from build123d import *

# Parameters (mm, degrees)
SKETCH_1_R               = 20
EXTRUDE_1_DEPTH          = 5
M3X0_5_1_D               = 2.5
M3X0_5_1_DEPTH           = 7.5
M3X0_5_1_TIP             = 0.751075774
SKETCH_6_R               = 12
EXTRUDE_2_DEPTH          = 30
SKETCH_7_R               = 10
CUT_EXTRUDE_2_DEPTH      = 30
CHAMFER_1_SIZE           = 0.5
CUT_EXTRUDE_3_DEPTH      = 46
CUT_EXTRUDE_3_DEPTH_BACK = 46
SKETCH_8_R               = 3
CHAMFER_2_SIZE           = 0.5
CHAMFER_3_SIZE           = 0.5


with BuildPart() as part:
    # 草图1 → 凸台-拉伸1 (new body)
    with BuildSketch(Plane(origin=(0, 0, 0), x_dir=(0, 0, -1), z_dir=(1, 0, 0))):
        Circle(SKETCH_1_R)
    extrude(amount=EXTRUDE_1_DEPTH)

    # M3x0.5 螺纹孔1
    with Locations(Plane.ZY):
        with Locations((-13.856406461, 8), (13.856406461, 8), (0, -16)):
            Hole(M3X0_5_1_D / 2, depth=M3X0_5_1_DEPTH)
            with Locations((0, 0, -(M3X0_5_1_DEPTH + M3X0_5_1_TIP / 2))):  # 118° drill point
                Cone(0, M3X0_5_1_D / 2, M3X0_5_1_TIP, mode=Mode.SUBTRACT)

    # 草图6 → 凸台-拉伸2 (add)
    with BuildSketch(Plane(origin=(5, 0, 0), x_dir=(0, 0, -1), z_dir=(1, 0, 0))):
        Circle(SKETCH_6_R)
    extrude(amount=EXTRUDE_2_DEPTH)

    # 草图7 → 切除-拉伸2 (cut)
    with BuildSketch(Plane(origin=(35, 0, 0), x_dir=(0, 0, -1), z_dir=(1, 0, 0))):
        Circle(SKETCH_7_R)
    extrude(amount=-CUT_EXTRUDE_2_DEPTH, mode=Mode.SUBTRACT)

    # 倒角1
    chamfer_1_edges = [part.edges().sort_by_distance(p)[0] for p in [
        (35, 0, 12),
    ]]
    chamfer(chamfer_1_edges, length=CHAMFER_1_SIZE)

    # 草图8 → 切除-拉伸3 (cut, two sides: drawn at the far end of the back side and taken through both)
    with BuildSketch(Plane(origin=(0, 0, 0), x_dir=(1, 0, 0), z_dir=(0, 1, 0)).offset(-CUT_EXTRUDE_3_DEPTH_BACK)):
        with Locations(Location((25, 0, 0), (0, 0, 90))):
            Circle(SKETCH_8_R)
    extrude(amount=CUT_EXTRUDE_3_DEPTH + CUT_EXTRUDE_3_DEPTH_BACK, mode=Mode.SUBTRACT)

    # 倒角2
    chamfer_2_edges = [part.edges().sort_by_distance(p)[0] for p in [
        (5, 0, 20),
    ]]
    chamfer(chamfer_2_edges, length=CHAMFER_2_SIZE)

    # 倒角3
    chamfer_3_edges = [part.edges().sort_by_distance(p)[0] for p in [
        (5, 0, 12),
    ]]
    chamfer(chamfer_3_edges, length=CHAMFER_3_SIZE)


solid = part.part
The listing builds one solid part. Answer for the finished solid, in the listing's coordinates (mm). A direction names the side the tool comes from. Give positions to 0.01 mm unless a question says otherwise; leave off trailing zeros. Write each loop counter-clockwise with the first axis right and the second up, starting at its lowest first coordinate (ties: lowest second). Pieces come first, ordered by that corner, then holes. Notation, with made-up numbers: (37.25, 34) - (73.25, 34) arc R10 cw to (73.25, 38) - close; hole circle Ø6 at (54.25, 57.5). An arc over 180 degrees is marked (long way). One line per question, with ' | ' between items. Start each with the question number.
1. Determine the mould class of faces 3 (the face through (5, 0, -13)), 4 (the face through (2.54, 6.89, 13.28)), 5 (the face through (5, 0, 0)), 6 (the face through (2.218, -19.524, 4.336)) for opening direction Z: +Z half, -Z half, draft (parallel to the pull), parting line (faces both ways), or undercut.
2. Section B-B, the plane x = 26.5 is taken. Determine the outline of the cut face in (y, z), then the cut area to 3 significant figures.
3. Section C-C, the plane y = 0 is taken. Determine the outline of the cut face in (x, z).
4. Section A-A, the plane z = 0 is taken. Count the separate pieces of the cut face and the enclosed holes in it, then the cut area to 3 significant figures.
5. Given P1, Ø1, axis at x = 23.5, y = 3.5, coming from the -Z side; P2, Ø3, axis at x = 12, y = 15, coming from the +Z side; P3, Ø1, axis at x = 28, y = 6.5, coming from the +Z side; P4, Ø3, axis at y = 8, z = -13.86, coming from the +X side, each flat-ended and moving along its own axis, determine where each tip first touches the part or whether it passes through.
6. Section D-D, the plane x = 14 is taken. Determine the outline of the cut face in (y, z), then the cut area to 3 significant figures.
7. Straight lines are drawn through the part: line 1 (Y direction, x = 11, z = -0.5); line 2 (X direction, y = 5, z = 0); line 3 (Z direction, x = 25, y = 10.9). For each, find the intervals that lie inside material, in ascending order.
8. For faces 1 (the face through (2.535, 8.055, -12.608)), 2 (the face through (20.21, 3, -9.54)), determine the directions among +Z, -Z, +X, -X, +Y, -Y from which every point of the face is accessible in a straight line to the end or side of a thin tool.
Result:
1) face 3: draft | face 4: undercut | face 5: undercut | face 6: parting line
2) outline: (-11.72, -2.6) arc R12 ccw to (11.72, -2.6) - (9.66, -2.6) arc R10 cw to (-9.66, -2.6) - close; (-11.72, 2.6) - (-9.66, 2.6) arc R10 cw to (9.66, 2.6) - (11.72, 2.6) arc R12 ccw to start | area: 117 mm2
3) outline: (0, -20) - (4.5, -20) - (5, -19.5) - (5, -12.5) - (5.5, -12) - (34.5, -12) - (35, -11.5) - (35, -10) - (5, -10) - (5, 10) - (35, 10) - (35, 11.5) - (34.5, 12) - (5.5, 12) - (5, 12.5) - (5, 19.5) - (4.5, 20) - (0, 20) - close
4) separate pieces: 4 | enclosed holes: 0 | area: 283 mm2
5) P1: stops at z = -11.62 | P2: passes through | P3: stops at z = 10.39 | P4: stops at x = 5
6) outline: circle Ø24 at (0, 0); hole circle Ø20 at (0, 0) | area: 138 mm2
7) line 1: y = -11.99 to -9.99, 9.99 to 11.99 | line 2: x = 0 to 5 | line 3: z = -5.02 to -3, 3 to 5.02
8) face 1: +X, -X | face 2: +X
